Could you check a few things on this model? Use its own coordinates, in mm. A direction names the side the tool comes from. Give positions to 0.01 mm unless a question says otherwise; leave off trailing zeros. Order: outer loops, then holes, each group sorted by start corner. A loop starts at its lowest first (then second) coordinate and runs counter-clockwise, first axis right, second up.
from build123d import *

# Parameters (mm, degrees)
SKETCH1_R           = 61
SKETCH1_R_2         = 56
BOSS_EXTRUDE1_DEPTH = 300
SKETCH3_R           = 56
BOSS_EXTRUDE2_DEPTH = 5
CUT_EXTRUDE1_REACH  = 294.988
SKETCH4_R           = 1.5
SKETCH5_R           = 56
BOSS_EXTRUDE3_DEPTH = 5
CUT_EXTRUDE2_REACH  = 299.77
SKETCH6_W           = 25.301187414
SKETCH6_H           = 10.224452448


with BuildPart() as part:
    # Sketch1 → Boss-Extrude1 (new body)
    with BuildSketch(Plane(origin=(0, 0, 0), x_dir=(1, 0, 0), z_dir=(0, 1, 0))):
        with Locations(Location((0, 0, 0), (0, 0, 270))):
            Circle(SKETCH1_R)
        with Locations(Location((0, 0, 0), (0, 0, 270))):
            Circle(SKETCH1_R_2, mode=Mode.SUBTRACT)
    extrude(amount=BOSS_EXTRUDE1_DEPTH)

    # Sketch3 → Boss-Extrude2 (add)
    with BuildSketch(Plane(origin=(0, 20, 0), x_dir=(1, 0, 0), z_dir=(0, 1, 0))):
        with Locations(Location((0, 0, 0), (0, 0, 270))):
            Circle(SKETCH3_R)
    extrude(amount=BOSS_EXTRUDE2_DEPTH)

    # Sketch4 → Cut-Extrude1 (cut, up to next)
    with BuildSketch(Plane.XZ.offset(-20), mode=Mode.PRIVATE) as cut_extrude1_sk1:
        with Locations(Location((-3, 0, 0), (0, 0, 270))):
            Circle(SKETCH4_R)
    cut_extrude1_tool1 = extrude(cut_extrude1_sk1.sketch, amount=-CUT_EXTRUDE1_REACH, mode=Mode.PRIVATE) & part.part
    # Sketch4 → Cut-Extrude1 (cut, up to next)
    with BuildSketch(Plane.XZ.offset(-20), mode=Mode.PRIVATE) as cut_extrude1_sk2:
        with Locations(Location((3, 0, 0), (0, 0, 270))):
            Circle(SKETCH4_R)
    cut_extrude1_tool2 = extrude(cut_extrude1_sk2.sketch, amount=-CUT_EXTRUDE1_REACH, mode=Mode.PRIVATE) & part.part
    add(cut_extrude1_tool1.solids().sort_by_distance((-3, 20, 0))[0], mode=Mode.SUBTRACT)
    add(cut_extrude1_tool2.solids().sort_by_distance((3, 20, 0))[0], mode=Mode.SUBTRACT)

    # Sketch5 → Boss-Extrude3 (add)
    with BuildSketch(Plane(origin=(0, 280, 0), x_dir=(1, 0, 0), z_dir=(0, 1, 0))):
        with Locations(Location((0, 0, 0), (0, 0, 270))):
            Circle(SKETCH5_R)
    extrude(amount=BOSS_EXTRUDE3_DEPTH)

    # Sketch6 → Cut-Extrude2 (cut, up to next)
    with BuildSketch(Plane(origin=(0, 285, 0), x_dir=(1, 0, 0), z_dir=(0, 1, 0)), mode=Mode.PRIVATE) as cut_extrude2_sk1:
        Rectangle(SKETCH6_W, SKETCH6_H)
    cut_extrude2_tool1 = extrude(cut_extrude2_sk1.sketch, amount=-CUT_EXTRUDE2_REACH, mode=Mode.PRIVATE) & part.part
    add(cut_extrude2_tool1.solids().sort_by_distance((0, 285, 0))[0], mode=Mode.SUBTRACT)


solid = part.part
Item 1: Imagine slicing it at B-B on z = 36. List the corners of the cut face in (x, y) for me.
Findings:
outline: (-49.24, 0) - (-42.9, 0) - (-42.9, 20) - (42.9, 20) - (42.9, 0) - (49.24, 0) - (49.24, 300) - (42.9, 300) - (42.9, 285) - (-42.9, 285) - (-42.9, 300) - (-49.24, 300) - close; hole (-42.9, 25) - (42.9, 25) - (42.9, 280) - (-42.9, 280) - close
Item 2: We'd pull the mould along X, two halves only. Please class faces 5 (the cylindrical face through (-59.55, 147.9, -13.22)), 6 (the flat face through (-26.8, 300, 49.4)), 7 (the cylindrical face through (-54.67, 292.4, -12.14)): +X half, -X half, draft (parallel to the pull), parting line (faces both ways), or undercut.
Findings:
face 5: parting line
face 6: draft
face 7: undercut
Item 3: Please list where these lines run through material, in increasing order: line 1 along X through (y, z) = (23.7, 0); line 2 along X through (y, z) = (240.5, -1); line 3 along Y through (x, z) = (-52.5, 3).
Findings:
line 1: x = -61 to -4.5, -1.5 to 1.5, 4.5 to 61
line 2: x = -60.99 to -55.99, 55.99 to 60.99
line 3: y = 20 to 25, 280 to 285
Item 4: Imagine slicing it at A-A on x = 17. List the corners of the cut face in (y, z) for me.
Findings:
outline: (0, -58.58) - (300, -58.58) - (300, -53.36) - (285, -53.36) - (285, 53.36) - (300, 53.36) - (300, 58.58) - (0, 58.58) - (0, 53.36) - (20, 53.36) - (20, -53.36) - (0, -53.36) - close; hole (25, -53.36) - (280, -53.36) - (280, 53.36) - (25, 53.36) - close
Item 5: For faces 1 (the cylindrical face through (-54.67, 150.72, -12.14)), 2 (the flat face through (1, 20, -1)), 3 (the flat face through (-26.8, 0, 49.4)), 4 (the flat face through (1, 285, 12)), which set-ups out of +Z, -Z, +X, -X, +Y, -Y let a thin tool reach every point of the face, with its end or its side?
Findings:
face 1: none
face 2: -Y
face 3: +Z, -Z, +X, -X, -Y
face 4: +Y
Item 6: For pin 1 (2 mm diameter, centred on y = 74, z = 13, fed in from +X); pin 2 (6 mm diameter, centred on y = 50.5, z = -32.5, fed in from -X); pin 3 (4 mm diameter, centred on x = -3, z = 0, fed in from -Y), each with a flat end and sliding along its axis, tell me the tip position at first contact or that it passes through.
Findings:
pin 1: stops at x = 59.81
pin 2: stops at x = -53.39
pin 3: stops at y = 20
Item 7: Imagine slicing it at C-C on y = 251. List the corners of the cut face in (x, z) for me, then the cut area to 3 significant figures.
Findings:
outline: circle Ø122 at (0, 0); hole circle Ø112 at (0, 0)
area: 1,840 mm2
